from build123d import *

# Parameters (mm, degrees)
F0_W        = 250
F0_H        = 198.5
F1_DEPTH    = 3
F2_W        = 235
F2_H        = 7.5
F3_DEPTH    = 30
F5_DEPTH    = 300
F6_T1_DEPTH = 17.7867319519
F6_T3_DEPTH = 17.7867319519
F8_DEPTH    = 25
F9_SIZE     = 2.99999
F10_R       = 1.05
F11_DEPTH   = 1.1


# Not quite as in the source:
# - a fillet or chamfer that OpenCascade refuses, or shapes differently, is made with other operations: its cross-section is extruded or revolved along the edge and cut away or added
# - a fillet or chamfer is up to 0.001 mm smaller than in the source, because OpenCascade refuses the exact size


with BuildPart() as f1:
    # F0 (on Front) → F1 (new body)
    with BuildSketch(Plane.XZ):
        Rectangle(F0_W, F0_H)
    extrude(amount=F1_DEPTH)

    # F2 (on face) → F3 (cut)
    with BuildSketch(Plane.XZ.offset(3)):
        with Locations((0, -95.5)):
            Rectangle(F2_W, F2_H)
    extrude(amount=-F3_DEPTH, mode=Mode.SUBTRACT)

    # F4 (on face) → F5 (cut)
    with BuildSketch(Plane.YZ.offset(-117.5)):
        with BuildLine():
            ThreePointArc((-1.25, -97.25), (-1.6767766953, -97.0732233047), (-1.5, -97.5))
            ThreePointArc((-1.5, -97.5), (-1.3232233047, -97.4267766953), (-1.25, -97.25))
        make_face()
    extrude(amount=-F5_DEPTH, mode=Mode.SUBTRACT)

    # F6: chamfer of 2 on 4 edges, made by hand

    # F6_s2 → F6_t1 (cut)
    with BuildSketch(Plane.YZ.offset(-130.1433659759)):
        Polygon((-3, -97.25), (-1, -99.25), (-3, -99.25), align=None)
        Polygon((0, -97.25), (-2, -99.25), (0, -99.25), align=None)
    extrude(amount=F6_T1_DEPTH, mode=Mode.SUBTRACT)

    # F6_s4 → F6_t3 (cut)
    with BuildSketch(Plane.YZ.offset(112.3566340241)):
        Polygon((-3, -97.25), (-1, -99.25), (-3, -99.25), align=None)
        Polygon((0, -97.25), (-2, -99.25), (0, -99.25), align=None)
    extrude(amount=F6_T3_DEPTH, mode=Mode.SUBTRACT)

    # F7 (on face) → F8 (cut)
    with BuildSketch(Plane.XZ.offset(3)):
        Polygon((0, 89.25), (-10.6066017178, 78.6433982822), (0, 68.0367965644), (10.6066017178, 78.6433982822), align=None)
    extrude(amount=-F8_DEPTH, mode=Mode.SUBTRACT)

    # F9 (size 3 in the source; OpenCascade refuses exactly that, so slightly less here)
    f9_edges = [f1.edges().sort_by_distance(p)[0] for p in [
        (0, -3, 99.25),
    ]]
    chamfer(f9_edges, length=F9_SIZE)

    # F10 (on face) → F11 (cut)
    with BuildSketch(Plane(origin=(0, 0, 0), x_dir=(-1, 0, 0), z_dir=(0, 1, 0))):
        with BuildLine():
            Line((-122.45, 93.25), (-123.5, 93.25))
            Line((-123.5, 93.25), (-124.55, 93.25))
            ThreePointArc((-124.55, 93.25), (-123.5, 92.2), (-122.45, 93.25))
        make_face()
        with BuildLine():
            Line((-123.5, 94.3), (-123.5, 93.25))
            Line((-123.5, 93.25), (-122.45, 93.25))
            ThreePointArc((-122.45, 93.25), (-122.7575378798, 93.9924621202), (-123.5, 94.3))
        make_face()
        with BuildLine():
            Line((-124.55, 93.25), (-123.5, 93.25))
            Line((-123.5, 93.25), (-123.5, 94.3))
            ThreePointArc((-123.5, 94.3), (-124.2424621202, 93.9924621202), (-124.55, 93.25))
        make_face()
        with Locations((123.5, 93.25)):
            Circle(F10_R)
    extrude(amount=-F11_DEPTH, mode=Mode.SUBTRACT)


solid = f1.part
Part model, mm, in its own coordinate system. A direction names the side the tool comes from. Give positions to 0.01 mm unless a question says otherwise; leave off trailing zeros. One line per question, with ' | ' between items.
1. Pull direction Z, two halves, no side cores. Call faces 1 (the face through (-5.23, -1.52, 84.02)), 2 (the face through (-2, 0, 2)): +Z half, -Z half, draft (parallel to the pull), parting line (faces both ways), or undercut.
Filled in:
face 1: undercut | face 2: draft
2. Drop flat-ended pins along their axis: P1, Ø1, axis at x = -73, y = -0.5, coming from the -Z side; P2, Ø2, axis at x = -4, z = 53, coming from the +Y side. Give the stop position or say it passes through.
Filled in:
P1: z = -91.75 | P2: y = 0
3. Drill centre lines: probe 1 along X at (y, z) = (-0.9, 93.25); probe 2 along X at (y, z) = (-0.25, 77); probe 3 along Z at (x, y) = (-120, -1.5). Where is each one in solid material? Low to high.
Filled in:
probe 1: -125 to -124.55, -122.45 to 122.45, 124.55 to 125 | probe 2: -125 to -8.96, 8.96 to 125 | probe 3: -98.75 to -97.5, -97 to 97.75
4. Which spindle directions (+Z, -Z, +X, -X, +Y, -Y) get a long thin tool onto all of the face, cutting with end or side? Do faces 3 (the face through (-5.378, -1.521, 73.414)), 4 (the face through (-2, -3, 1)). Say none if no direction does.
Filled in:
face 3: +Y, -Y | face 4: +Z, -Z, +X, -X, -Y
